```python
from build123d import *

# Parameters (mm, degrees)
EXTRUDE1_DEPTH                               = 200
FILLET1_R                                    = 0.5
CSK_FOR_M4_COUNTERSUNK_FLAT_HEAD_SCR_2_COUNT = 2
CSK_FOR_M4_COUNTERSUNK_FLAT_HEAD_SCR_2_PITCH = 45
CSK_FOR_M3_COUNTERSUNK_FLAT_HEAD_SCR_2_COUNT = 2
CSK_FOR_M3_COUNTERSUNK_FLAT_HEAD_SCR_2_PITCH = 15
CSK_FOR_M3_COUNTERSUNK_FLAT_HEAD_SCR_3_COUNT = 2
CSK_FOR_M3_COUNTERSUNK_FLAT_HEAD_SCR_3_PITCH = 15
M3_TAPPED_HOLE1_D                            = 3
M3_TAPPED_HOLE1_DEPTH                        = 2.001
LPATTERN1_COUNT                              = 6
LPATTERN1_PITCH                              = 38.4


with BuildPart() as part:
    # Sketch1 → Extrude1 (new body)
    with BuildSketch(Plane.XY):
        Polygon((0, 0), (0, 28), (-28, 28), (-28, 30), (2, 30), (2, 0), align=None)
    extrude(amount=EXTRUDE1_DEPTH)

    # Fillet1
    fillet1_edges = [part.edges().sort_by_distance(p)[0] for p in [
        (-28, 28, 100),
        (-28, 30, 100),
        (2, 30, 100),
        (2, 0, 100),
        (0, 0, 100),
    ]]
    fillet(fillet1_edges, radius=FILLET1_R)

    # Sketch4 → CSK for M4 Countersunk Flat Head Screw1 (revolve, cut)
    with BuildSketch(Plane(origin=(-5, 30, 69), x_dir=(0, 0, 1), z_dir=(1, 0, 0))):
        Polygon((0, 0), (0, 2), (2.25, 2), (2.25, 2.45), (4.7, 0), align=None)
    csk_for_m4_countersunk_flat_head_screw1 = revolve(axis=Axis((-5, 36.35, 69), (0, -1, 0)), mode=Mode.SUBTRACT)

    # CSK for M4 Countersunk Flat Head Scr 2: CSK for M4 Countersunk Flat Head Screw1 ×2
    with Locations(*[(0, 0, -i * CSK_FOR_M4_COUNTERSUNK_FLAT_HEAD_SCR_2_PITCH) for i in range(1, CSK_FOR_M4_COUNTERSUNK_FLAT_HEAD_SCR_2_COUNT)]):
        add(csk_for_m4_countersunk_flat_head_screw1, mode=Mode.SUBTRACT)

    # Sketch5 → CSK for M3 Countersunk Flat Head Screw1 (revolve, cut)
    with BuildSketch(Plane(origin=(-19, 30, 4), x_dir=(0, 0, 1), z_dir=(1, 0, 0))):
        Polygon((0, 0), (0, 2), (1.7, 2), (1.7, 1.45), (3.15, 0), align=None)
    csk_for_m3_countersunk_flat_head_screw1 = revolve(axis=Axis((-19, 36.35, 4), (0, -1, 0)), mode=Mode.SUBTRACT)

    # CSK for M3 Countersunk Flat Head Scr 2: CSK for M3 Countersunk Flat Head Screw1 ×2
    with Locations(*[(i * CSK_FOR_M3_COUNTERSUNK_FLAT_HEAD_SCR_2_PITCH, 0, 0) for i in range(1, CSK_FOR_M3_COUNTERSUNK_FLAT_HEAD_SCR_2_COUNT)]):
        add(csk_for_m3_countersunk_flat_head_screw1, mode=Mode.SUBTRACT)

    # Sketch6 → CSK for M3 Countersunk Flat Head Screw2 (revolve, cut)
    with BuildSketch(Plane(origin=(-19, 30, 196), x_dir=(0, 0, 1), z_dir=(1, 0, 0))):
        Polygon((0, 0), (0, 2), (1.7, 2), (1.7, 1.45), (3.15, 0), align=None)
    csk_for_m3_countersunk_flat_head_screw2 = revolve(axis=Axis((-19, 36.35, 196), (0, -1, 0)), mode=Mode.SUBTRACT)

    # CSK for M3 Countersunk Flat Head Scr 3: CSK for M3 Countersunk Flat Head Screw2 ×2
    with Locations(*[(i * CSK_FOR_M3_COUNTERSUNK_FLAT_HEAD_SCR_3_PITCH, 0, 0) for i in range(1, CSK_FOR_M3_COUNTERSUNK_FLAT_HEAD_SCR_3_COUNT)]):
        add(csk_for_m3_countersunk_flat_head_screw2, mode=Mode.SUBTRACT)

    # M3 Tapped Hole1
    with Locations(Plane(origin=(2, 24, 4), x_dir=(0, 1, 0), z_dir=(1, 0, 0))):
        with Locations((0, 0)):
            m3_tapped_hole1 = Hole(M3_TAPPED_HOLE1_D / 2, depth=M3_TAPPED_HOLE1_DEPTH)

    # LPattern1: M3 Tapped Hole1 ×6
    with Locations(*[(0, 0, i * LPATTERN1_PITCH) for i in range(1, LPATTERN1_COUNT)]):
        add(m3_tapped_hole1, mode=Mode.SUBTRACT)


solid = part.part
```
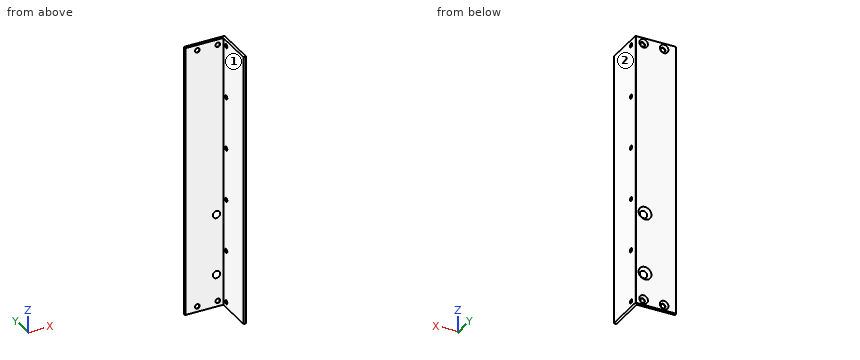
Model file for the job. Use its own axes, mm. Face numbers are marked on the shaded views. A direction names the side the tool comes from. Round coordinates to 2 decimals unless told otherwise and drop trailing zeros. Write each loop counter-clockwise with the first axis right and the second up, starting at its lowest first coordinate (ties: lowest second). Pieces come first, ordered by that corner, then holes. Notation, with made-up numbers: (83.5, -5.5) -> (137.5, -5.5) arc R16 ccw to (137.5, 0.5) -> close; hole circle Ø7 at (48, -28.75). An arc over 180 degrees is marked (long way). Answer as CSV lines item,"result".
1. Slice it at A-A, the plane z = 24. List the corners of the cut face in (x, y).
Resolved:
outline,"(-28, 28.5) arc R0.5 ccw to (-27.5, 28) -> (-7.7, 28) -> (-9.7, 30) -> (-27.5, 30) arc R0.5 ccw to (-28, 29.5) -> close; (-2.3, 28) -> (0, 28) -> (0, 0.5) arc R0.5 ccw to (0.5, 0) -> (1.5, 0) arc R0.5 ccw to (2, 0.5) -> (2, 29.5) arc R0.5 ccw to (1.5, 30) -> (-0.3, 30) -> close"
2. Slice it at B-B, the plane z = 91.5. List the corners of the cut face in (x, y), plus the area to 3 significant figures.
Resolved:
outline,"(-28, 28.5) arc R0.5 ccw to (-27.5, 28) -> (0, 28) -> (0, 0.5) arc R0.5 ccw to (0.5, 0) -> (1.5, 0) arc R0.5 ccw to (2, 0.5) -> (2, 29.5) arc R0.5 ccw to (1.5, 30) -> (-27.5, 30) arc R0.5 ccw to (-28, 29.5) -> close"
area,"116 mm²"
3. Drill centre lines: line 1 (X direction, y = 28.45, z = 196); line 2 (Y direction, x = 0.5, z = 80.8); line 3 (X direction, y = 7.5, z = 49). Where is each one in solid material? Low to high.
Resolved:
line 1,"-28 to -20.7, -17.3 to -5.7, -2.3 to 2"
line 2,"0 to 22.5, 25.5 to 30"
line 3,"0 to 2"
4. Pin check, flat tips, straight feed: pin 1 Ø4 at (x, y) = (-24, 25.5) entering from +Z; pin 2 Ø8 at (y, z) = (16.5, 58.5) entering from -X; pin 3 Ø1 at (x, z) = (-18.5, 166.5) entering from -Y. Stop position of each tip, or through.
Resolved:
pin 1,"through"
pin 2,"x = 0"
pin 3,"y = 28"
5. Tool access for the marked faces 1 and 2: list every direction of +Z, -Z, +X, -X, +Y, -Y with a clear straight run to the whole face (end or side of a thin tool).
Resolved:
face 1,"+Z, -Z, -X, -Y"
face 2,"+Z, -Z, +X, +Y, -Y"
6. Slice it at D-D, the plane y = 20.5. List the corners of the cut face in (x, z), plus the area to 3 significant figures.
Resolved:
outline,"(0, 0) -> (2, 0) -> (2, 200) -> (0, 200) -> close"
area,"400 mm²"
7. Slice it at C-C, the plane x = -12.25. List the corners of the cut face in (y, z), plus the area to 3 significant figures.
Resolved:
outline,"(28, 0) -> (30, 0) -> (30, 200) -> (28, 200) -> close"
area,"400 mm²"
